from build123d import *

# Parameters (mm, degrees)
SKETCH1_R           = 2
BOSS_EXTRUDE2_DEPTH = 10
SKETCH2_R           = 2
CUT_EXTRUDE1_DEPTH  = 87.986099448


with BuildPart() as part:
    # Sketch1 → Boss-Extrude2 (new body)
    with BuildSketch(Plane(origin=(0, 0, 0), x_dir=(1, 0, 0), z_dir=(0, 1, 0))):
        with BuildLine():
            Line((-76.197237464, -6.35), (-36.197237464, -6.35))
            ThreePointArc((-36.197237464, -6.35), (1.186838378, -36.730830574), (36.531664348, -4))
            Line((36.531664348, -4), (46.531664348, -4))
            Line((46.531664348, -4), (46.531664348, -0.5))
            Line((46.531664348, -0.5), (28.745651845, -0.5))
            ThreePointArc((28.745651845, -0.5), (-28.75, 0), (28.745651845, 0.5))
            Line((28.745651845, 0.5), (46.531664348, 0.5))
            Line((46.531664348, 0.5), (46.531664348, 4))
            Line((46.531664348, 4), (36.531664348, 4))
            ThreePointArc((36.531664348, 4), (1.186838378, 36.730830574), (-36.197237464, 6.35))
            Line((-36.197237464, 6.35), (-76.197237464, 6.35))
            Line((-76.197237464, 6.35), (-76.197237464, -6.35))
        make_face()
        with Locations(Location((-69.197237464, 0, 0), (0, 0, 270))):
            Circle(SKETCH1_R, mode=Mode.SUBTRACT)
        with Locations(Location((-54.197237464, 0, 0), (0, 0, 270))):
            Circle(SKETCH1_R, mode=Mode.SUBTRACT)
    extrude(amount=BOSS_EXTRUDE2_DEPTH)

    # Sketch2 → Cut-Extrude1 (cut, through all)
    with BuildSketch(Plane.XY.offset(4)):
        with Locations((41.531664348, 5)):
            Circle(SKETCH2_R)
    extrude(amount=-CUT_EXTRUDE1_DEPTH, mode=Mode.SUBTRACT)


solid = part.part
Part model, mm, in its own coordinate system. A direction names the side the tool comes from. Coordinates: 2 decimals unless noted, no trailing zeros. Loops run counter-clockwise (first coordinate to the right, second up) from the corner with the lowest first, then second, coordinate; pieces in that order, holes last. Notation, with made-up numbers: (-34.5, 20.25) - (5.5, 20.25) arc R30 cw to (5.5, 59.25) - close; hole circle Ø11 at (18.5, -1). An arc over 180 degrees is marked (long way). Write each question's results on one line, items separated by ' | '. Start each with the question number.
Q1. Two-plate mould, pull along Z, no slides. Class faces 1 (the flat face through (46.532, 5, 2)), 2 (the cylindrical face through (-55.972, 4.93, 0.923)), 3 (the cylindrical face through (0.452, 4.93, 36.747)): +Z half, -Z half, draft (parallel to the pull), parting line (faces both ways), or undercut.
Q2. Drop flat-ended pins along their axis: pin 1 Ø4 at (y, z) = (8, -26) entering from +X; pin 2 Ø4.5 at (x, y) = (41.53, 5) entering from -Z; pin 3 Ø4.5 at (x, y) = (41.53, 5) entering from +Z. Give the stop position or say it passes through.
Q3. Slice it at C-C on y = 5. Give the cut face in (x, z), and give its area (3 significant figures).
Q4. Probe line 1 along X through (y, z) = (5, 0); line 2 along Z through (x, y) = (41, 0.75); line 3 along Z through (x, y) = (-42.5, 7.5). List the from-to ranges inside material, lowest first.
Q5. Slice it at D-D on x = -49. Give the cut face in (y, z).
Q6. Which spindle directions (+Z, -Z, +X, -X, +Y, -Y) get a long thin tool onto all of the face, cutting with end or side? Do faces 4 (the flat face through (39, 5, -4)), 5 (the flat face through (38, 5, -0.5)), 6 (the flat face through (-56, 5, 6.35)). Say none if no direction does.
Q7. Slice it at B-B on z = -19. Give the cut face in (x, y), and give its area (3 significant figures).
Q8. Slice it at A-A on x = 0. Give the cut face in (y, z).
Answer:
1) face 1: draft | face 2: undercut | face 3: +Z half
2) pin 1: stops at x = 27.83 | pin 2: stops at z = -4 | pin 3: stops at z = 4
3) outline: (-76.2, -6.35) - (-36.2, -6.35) arc R36.75 ccw to (36.53, -4) - (39.53, -4) - (39.53, -0.5) - (28.75, -0.5) arc R28.75 cw (long way) to (28.75, 0.5) - (39.53, 0.5) - (39.53, 4) - (36.53, 4) arc R36.75 ccw to (-36.2, 6.35) - (-76.2, 6.35) - close; (43.53, -4) - (46.53, -4) - (46.53, -0.5) - (43.53, -0.5) - close; (43.53, 0.5) - (46.53, 0.5) - (46.53, 4) - (43.53, 4) - close; hole circle Ø4 at (-69.2, 0); hole circle Ø4 at (-54.2, 0) | area: 2,160 mm2
4) line 1: x = -76.2 to -71.2, -67.2 to -56.2, -52.2 to -28.75 | line 2: z = -4 to -0.5, 0.5 to 4 | line 3: z = -6.35 to 6.35
5) outline: (0, -6.35) - (10, -6.35) - (10, 6.35) - (0, 6.35) - close
6) face 4: -Z, +X, +Y, -Y | face 5: +X, +Y, -Y | face 6: +Z, -X, +Y, -Y
7) outline: (-31.46, 0) - (-21.58, 0) - (-21.58, 10) - (-31.46, 10) - close; (21.58, 0) - (31.46, 0) - (31.46, 10) - (21.58, 10) - close | area: 198 mm2
8) outline: (0, -36.75) - (10, -36.75) - (10, -28.75) - (0, -28.75) - close; (0, 28.75) - (10, 28.75) - (10, 36.75) - (0, 36.75) - close
